The model under review builds one solid part; all positions refer to its coordinate system, in mm. Face numbers are marked on the shaded views. A direction names the side the tool comes from. Coordinates: 2 decimals unless noted, no trailing zeros. Order: outer loops, then holes, each group sorted by start corner. A loop starts at its lowest first (then second) coordinate and runs counter-clockwise, first axis right, second up.
```python
from build123d import *

# Parameters (mm, degrees)
SKETCH2_R                           = 35
BOSS_EXTRUDE2_DEPTH                 = 30
SKETCH4_R                           = 43
BOSS_EXTRUDE3_DEPTH                 = 10
FILLET2_R                           = 10
SKETCH6_W                           = 10
SKETCH6_H                           = 30
EXTRUDE_THIN2_DEPTH                 = 15
SKETCH10_W                          = 10
SKETCH10_H                          = 15
BOSS_EXTRUDE4_DEPTH                 = 30
SKETCH11_W                          = 10
SKETCH11_H                          = 15
BOSS_EXTRUDE5_DEPTH                 = 30
FILLET4_R                           = 1
FILLET5_R                           = 0.5
CUT_EXTRUDE1_DEPTH                  = 127.256815818
CUT_EXTRUDE1_DEPTH_BACK             = 39
SKETCH12_W                          = 7.5
SKETCH12_H                          = 15
CUT_EXTRUDE2_REACH                  = 96.008
SKETCH17_W                          = 7.5
SKETCH17_H                          = 15
CUT_EXTRUDE3_DEPTH                  = 29
CUT_EXTRUDE3_DIRECTION_2_REACH      = 118.906
CUT_EXTRUDE3_DIRECTION_2_END_RADIUS = 7.5
CUT_EXTRUDE4_DEPTH                  = 1.25
SKETCH20_R                          = 2
CUT_EXTRUDE5_DEPTH                  = 1.25
CUT_EXTRUDE7_DEPTH                  = 1.25
SKETCH22_R                          = 5.25
CUT_EXTRUDE8_DEPTH                  = 1.25


with BuildPart() as part:
    # Sketch2 → Boss-Extrude2 (new body)
    with BuildSketch(Plane(origin=(0, 0, 0), x_dir=(1, 0, 0), z_dir=(0, 1, 0))):
        with Locations(Location((0, 0, 0), (0, 0, 270))):
            Circle(SKETCH2_R)
    extrude(amount=BOSS_EXTRUDE2_DEPTH)

    # Sketch4 → Boss-Extrude3 (add)
    with BuildSketch(Plane(origin=(0, 30, 0), x_dir=(1, 0, 0), z_dir=(0, 1, 0))):
        with Locations(Location((0, 0, 0), (0, 0, 270))):
            Circle(SKETCH4_R)
    extrude(amount=BOSS_EXTRUDE3_DEPTH)

    # Fillet2
    # the kernel refuses this fillet: 10 mm, written as the material it takes off along each edge
    with BuildSketch(Plane(origin=(0, 30, 0), x_dir=(0, 0, 1), z_dir=(-1, 0, 0))) as fillet2_piece_1:
        with BuildLine():
            CenterArc((33, 9.797958971), FILLET2_R, 281.536959033, 78.463040967)
            Line((35, 0), (35.04, -0.195959179))
            ThreePointArc((35.04, -0.195959179), (39, -0.2), (43, -0.2))
            Line((43, -0.2), (43.2, 0))
            Line((43.2, 0), (43.2, 9.797958971))
            Line((43.2, 9.797958971), (43, 9.797958971))
        make_face()
    revolve(axis=Axis((0, 30, 0), (0, 1, 0)), mode=Mode.SUBTRACT)

    # Sketch6 → Extrude-Thin2 (add)
    with BuildSketch(Plane(origin=(0, 0, 0), x_dir=(1, 0, 0), z_dir=(0, 0.7071067811865464, -0.7071067811865488))):
        with Locations((17, 15)):
            Rectangle(SKETCH6_W, SKETCH6_H)
        with Locations((-17, 15)):
            Rectangle(SKETCH6_W, SKETCH6_H)
    extrude(amount=EXTRUDE_THIN2_DEPTH)

    # Sketch10 → Boss-Extrude4 (add)
    with BuildSketch(Plane(origin=(0, -21.213203436, -21.213203436), x_dir=(1, 0, 0), z_dir=(0, -0.7071067811865487, -0.7071067811865465))):
        with Locations((17, -7.5)):
            Rectangle(SKETCH10_W, SKETCH10_H)
    extrude(amount=BOSS_EXTRUDE4_DEPTH)

    # Sketch11 → Boss-Extrude5 (add)
    with BuildSketch(Plane(origin=(0, -21.213203436, -21.213203436), x_dir=(1, 0, 0), z_dir=(0, -0.7071067811865487, -0.7071067811865465))):
        with Locations((-17, -7.5)):
            Rectangle(SKETCH11_W, SKETCH11_H)
    extrude(amount=BOSS_EXTRUDE5_DEPTH)

    # Fillet4
    fillet4_edges = [part.edges().sort_by_distance(p)[0] for p in [
        (-12, 0, -10.606601718),
        (-17, 0, -21.213203436),
        (-22, 0, -10.606601718),
        (-17, 0, 0),
        (12, 0, -10.606601718),
        (22, 0, -10.606601718),
        (17, 0, -21.213203436),
        (17, 0, 0),
    ]]
    fillet(fillet4_edges, radius=FILLET4_R)

    # Fillet5
    fillet5_edges = [part.edges().sort_by_distance(p)[0] for p in [
        (0, 0, -35),
    ]]
    fillet(fillet5_edges, radius=FILLET5_R)

    # Sketch12 → Cut-Extrude1 (cut, two sides: drawn at the far end of the back side and taken through both)
    with BuildSketch(Plane(origin=(0, -42.426406871, -42.426406871), x_dir=(1, 0, 0), z_dir=(0, -0.7071067811865485, -0.7071067811865467)).offset(-CUT_EXTRUDE1_DEPTH_BACK)):
        with Locations((-15.75, -7.5)):
            Rectangle(SKETCH12_W, SKETCH12_H)
    extrude(amount=CUT_EXTRUDE1_DEPTH + CUT_EXTRUDE1_DEPTH_BACK, mode=Mode.SUBTRACT)

    # Sketch13 → Cut-Extrude2 (cut, up to next)
    with BuildSketch(Plane.ZY.offset(22), mode=Mode.PRIVATE) as cut_extrude2_sk1:
        with BuildLine():
            Line((-42.426406871, -42.426406871), (-53.033008589, -31.819805153))
            Line((-53.033008589, -31.819805153), (-45.961940777, -24.748737342))
            ThreePointArc((-45.961940777, -24.748737342), (-45.961940777, -35.355339059), (-35.355339059, -35.355339059))
            Line((-35.355339059, -35.355339059), (-42.426406871, -42.426406871))
        make_face()
    cut_extrude2_tool1 = extrude(cut_extrude2_sk1.sketch, amount=-CUT_EXTRUDE2_REACH, mode=Mode.PRIVATE) & part.part
    add(cut_extrude2_tool1.solids().sort_by_distance((-22, -35.429094, -46.035696))[0], mode=Mode.SUBTRACT)
    add(cut_extrude2_tool1.solids().sort_by_distance((-22, -35.429094, -46.035696))[1], mode=Mode.SUBTRACT)

    # Sketch17 → Cut-Extrude3 (cut)
    with BuildSketch(Plane(origin=(0, -35.355339059, -35.355339059), x_dir=(-1, 0, 0), z_dir=(0, -0.7071067811865487, -0.7071067811865465))):
        with Locations((-15.75, 7.5)):
            Rectangle(SKETCH17_W, SKETCH17_H)
    extrude(amount=-CUT_EXTRUDE3_DEPTH, mode=Mode.SUBTRACT)

    # Cut-Extrude3 direction 2: up to this cylinder (the profile starts inside it)
    cut_extrude3_direction_2_end = Plane(origin=(15.75, -30.0520382, -40.658639918), z_dir=(-1, 0, 0)) * Cylinder(CUT_EXTRUDE3_DIRECTION_2_END_RADIUS, 253.812, mode=Mode.PRIVATE)
    # Sketch17 → Cut-Extrude3 direction 2 (cut, up to the surface)
    with BuildSketch(Plane(origin=(0, -35.355339059, -35.355339059), x_dir=(-1, 0, 0), z_dir=(0, -0.7071067811865487, -0.7071067811865465)), mode=Mode.PRIVATE) as cut_extrude3_direction_2_sk1:
        with Locations((-15.75, 7.5)):
            Rectangle(SKETCH17_W, SKETCH17_H)
    cut_extrude3_direction_2_tool1 = extrude(cut_extrude3_direction_2_sk1.sketch, amount=CUT_EXTRUDE3_DIRECTION_2_REACH, mode=Mode.PRIVATE) & cut_extrude3_direction_2_end
    add(cut_extrude3_direction_2_tool1.solids().sort_by_distance((15.75, -30.052038, -40.65864))[0], mode=Mode.SUBTRACT)

    # Sketch18 → Cut-Extrude4 (cut)
    with BuildSketch(Plane.ZY.offset(22)):
        Polygon((-44.309999675, -30.896234088), (-41.753224712, -33.636306452), (-38.101864956, -32.792110564), (-37.007280162, -29.207842313), (-39.564055124, -26.467769949), (-43.215414881, -27.311965837), align=None)
    extrude(amount=-CUT_EXTRUDE4_DEPTH, mode=Mode.SUBTRACT)

    # Sketch20 → Cut-Extrude5 (cut)
    with BuildSketch(Plane.ZY.offset(20.75)):
        with Locations((-40.658639918, -30.0520382)):
            Circle(SKETCH20_R)
    extrude(amount=-CUT_EXTRUDE5_DEPTH, mode=Mode.SUBTRACT)

    # Sketch21 → Cut-Extrude7 (cut)
    with BuildSketch(Plane(origin=(22, 0, 0), x_dir=(0, 0, -1), z_dir=(1, 0, 0))):
        Polygon((34.441125497, -28.162247172), (35.913275669, -34.491668124), (42.130790091, -36.381459152), (46.876154339, -31.941829228), (45.404004167, -25.612408277), (39.186489746, -23.722617249), align=None)
    extrude(amount=-CUT_EXTRUDE7_DEPTH, mode=Mode.SUBTRACT)

    # Sketch22 → Cut-Extrude8 (cut)
    with BuildSketch(Plane(origin=(20.75, 0, 0), x_dir=(0, 0, -1), z_dir=(1, 0, 0))):
        with Locations((40.658639918, -30.0520382)):
            Circle(SKETCH22_R)
    extrude(amount=-CUT_EXTRUDE8_DEPTH, mode=Mode.SUBTRACT)


solid = part.part
```
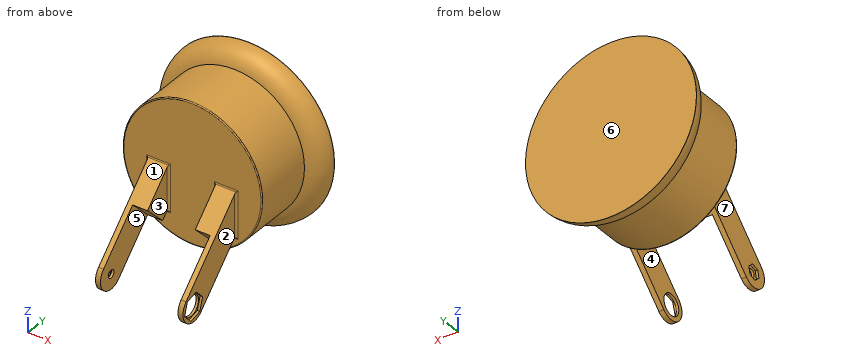
(1) Draft analysis for pull direction X (two halves, no side actions). For the marked faces 5, 6 and 7, state which applies: released by +X, released by -X, zero draft, split by the parting line, or undercut.
A:
face 5: undercut
face 6: zero draft
face 7: released by -X
(2) For pin 1 Ø2 at (y, z) = (-28.5, -40.5) entering from -X; pin 2 Ø13.5 at (y, z) = (-30.05, -40.66) entering from +X; pin 3 Ø2 at (x, z) = (-24, -29) entering from -Y, all flat-tipped, find the tip position at first contact; note any pin that passes through.
A:
pin 1: stops at x = -20.75
pin 2: stops at x = 22
pin 3: stops at y = 30.49
(3) We need section A-A, the plane x = 0. Write out the cut boundary in (y, z).
A:
outline: (0, -34.5) arc R0.5 ccw to (0.5, -35) - (30, -35) arc R10 ccw to (39.8, -43) - (40, -43) - (40, 43) - (39.8, 43) arc R10 ccw to (30, 35) - (0.5, 35) arc R0.5 ccw to (0, 34.5) - close
(4) Wall thickness on probe 1 along Y at (x, z) = (33, -9.5); probe 2 along X at (y, z) = (14, -1); probe 3 along Y at (x, z) = (-15.5, -19): over which ranges is each line inside the solid? List them lowest first.
A:
probe 1: y = 0 to 40
probe 2: x = -34.99 to 34.99
probe 3: y = -10.7 to 40
(5) We need section C-C, the plane y = 33. Write out the cut boundary in (x, z), and give its area (3 significant figures).
A:
outline: circle Ø80.67 at (0, 0)
area: 5,110 mm2
(6) Machinability: for the marked faces 1, 2, 3 and 4, which of the approach directions +Z, -Z, +X, -X, +Y, -Y give a long, thin tool a straight path to every point of the face, cutting with its end or side? Answer none if there is none.
A:
face 1: +Z, +X, -X, -Y
face 2: +Z, -Z, +X, -Y
face 3: +Z, -Z, -Y
face 4: -Z, -Y
(7) We need section B-B, the plane y = 16. Write out the cut boundary in (x, z).
A:
outline: circle Ø70 at (0, 0)
